CAD build for the part. Positions are in the model's coordinates, mm. A direction names the side the tool comes from. Round coordinates to 2 decimals unless told otherwise and drop trailing zeros. Loops run counter-clockwise (first coordinate to the right, second up) from the corner with the lowest first, then second, coordinate; pieces in that order, holes last. Notation, with made-up numbers: M 23,-35 L 43,-35 A14 ccw 43,-29 Z; hole C 62,20.5 d8. An arc over 180 degrees is marked long. Use a Markdown table: item, result. Add a question column.
(1) Which spindle directions (+Z, -Z, +X, -X, +Y, -Y) get a long thin tool onto all of the face, cutting with end or side? Do faces 4 (the face through (18, 91, 3)), 5 (the face through (8, -2, 3)), 6 (the face through (12.72, 107.75, 2.46)). Say none if no direction does.
(2) Band-saw the part on A-A, the plane y = 95. Write the cut outline in (x, z).
(3) Band-saw the part on D-D, the plane y = 70. Write the cut outline in (x, z), and give its area (3 significant figures).
(4) Flat gauge pins, fed straight in: P1, Ø13, axis at x = 16, y = 65, coming from the -Z side; P2, Ø0.9, axis at y = 105, z = 1.5, coming from the +X side. Where does each tip first touch, or does it go through?
(5) Two-plate mould, pull along Y, no slides. Class faces 1 (the face through (12.78, 102.25, 2.46)), 2 (the face through (11, 56, 0)), 3 (the face through (17.4, 111.43, 2.46)): released by +Y, released by -Y, zero draft, split by the parting line, or undercut.
(6) Band-saw the part on B-B, the plane x = 10. Write the cut outline in (y, z), and give its area (3 significant figures).
(7) Band-saw the part on C-C, the plane z = 1.45. Give the number of separate pieces and of enclosed holes in the cut face, and give its area (3 significant figures).
(8) Wall check: L1, parallel to Y at x = 10, z = 2.45; L2, parallel to Y at x = 2.5, z = 1.65; L3, parallel to Y at x = 4.25, z = 2.4. Give the ranges that are in metal, low to high.
from build123d import *

# Parameters (mm, degrees)
SKETCH1_W           = 24
SKETCH1_H           = 110
SKETCH1_R           = 4
SKETCH1_R_2         = 1.5
BOSS_EXTRUDE1_DEPTH = 5
SKETCH2_W           = 6
SKETCH2_H           = 37
SKETCH2_H_2         = 17
CUT_EXTRUDE1_DEPTH  = 113.698713391
BOSS_EXTRUDE2_DEPTH = 5
SKETCH4_R           = 1.5
SKETCH4_W           = 5
SKETCH4_H           = 10
CUT_EXTRUDE2_DEPTH  = 115.651646303
FILLET1_R           = 2
FILLET2_R           = 8


with BuildPart() as part:
    # Sketch1 → Boss-Extrude1 (new body)
    with BuildSketch(Plane.XY):
        with Locations((12, 55)):
            Rectangle(SKETCH1_W, SKETCH1_H)
        with Locations((16, 65)):
            Circle(SKETCH1_R, mode=Mode.SUBTRACT)
        with Locations((16, 25)):
            Circle(SKETCH1_R, mode=Mode.SUBTRACT)
        with Locations((10, 12)):
            Circle(SKETCH1_R_2, mode=Mode.SUBTRACT)
        with Locations((10, 95)):
            Circle(SKETCH1_R_2, mode=Mode.SUBTRACT)
        with BuildLine():
            Line((4, 103.5), (4, 106.5))
            ThreePointArc((4, 106.5), (5.25, 107.75), (6.5, 106.5))
            Line((6.5, 106.5), (6.5, 103.5))
            ThreePointArc((6.5, 103.5), (5.25, 102.25), (4, 103.5))
        make_face(mode=Mode.SUBTRACT)
        with BuildLine():
            Line((11.5, 103.5), (11.5, 106.5))
            ThreePointArc((11.5, 106.5), (12.75, 107.75), (14, 106.5))
            Line((14, 106.5), (14, 103.5))
            ThreePointArc((14, 103.5), (12.75, 102.25), (11.5, 103.5))
        make_face(mode=Mode.SUBTRACT)
    extrude(amount=BOSS_EXTRUDE1_DEPTH)

    # Sketch2 → Cut-Extrude1 (cut, through all)
    with BuildSketch(Plane.XY.offset(5)):
        with Locations((21, 91.5)):
            Rectangle(SKETCH2_W, SKETCH2_H)
        with Locations((21, 8.5)):
            Rectangle(SKETCH2_W, SKETCH2_H_2)
    extrude(amount=-CUT_EXTRUDE1_DEPTH, mode=Mode.SUBTRACT)

    # Sketch3 → Boss-Extrude2 (add)
    with BuildSketch(Plane.XY.offset(5)):
        Polygon((18, -2), (18, 0), (0, 0), (0, 110), (18, 110), (18, 112), (-2, 112), (-2, -2), align=None)
    extrude(amount=-BOSS_EXTRUDE2_DEPTH)

    # Sketch4 → Cut-Extrude2 (cut, through all)
    with BuildSketch(Plane.XY.offset(5)):
        with Locations((2.5, 20)):
            Circle(SKETCH4_R)
        with Locations((2.5, 70)):
            Circle(SKETCH4_R)
        with Locations((2.5, 5)):
            Rectangle(SKETCH4_W, SKETCH4_H)
        with Locations((2.5, 85)):
            Rectangle(SKETCH4_W, SKETCH4_H)
        with Locations((2.5, 45)):
            Rectangle(SKETCH4_W, SKETCH4_H)
    extrude(amount=-CUT_EXTRUDE2_DEPTH, mode=Mode.SUBTRACT)

    # Fillet1
    fillet1_edges = [part.edges().sort_by_distance(p)[0] for p in [
        (18, 112, 2.5),
        (-2, 112, 2.5),
        (-2, -2, 2.5),
        (18, -2, 2.5),
    ]]
    fillet(fillet1_edges, radius=FILLET1_R)

    # Fillet2
    # the kernel refuses this fillet: 8 mm, written as the material it takes off along each edge
    with BuildSketch(Plane(origin=(24, 17, 24.364916731), x_dir=(0, 1, 0), z_dir=(0, 0, -1))) as fillet2_piece_1:
        with BuildLine():
            CenterArc((7.745966692, -8), FILLET2_R, 90, 75.522487814)
            Line((0, -6), (-0.154919334, -5.96))
            ThreePointArc((-0.154919334, -5.96), (-0.16, -3), (-0.16, 0))
            Line((-0.16, 0), (0, 0.16))
            Line((0, 0.16), (7.745966692, 0.16))
            Line((7.745966692, 0.16), (7.745966692, 0))
        make_face()
    extrude(amount=43.729833462, mode=Mode.SUBTRACT)
    with BuildSketch(Plane(origin=(24, 73, 24.364916731), x_dir=(-1, 0, 0), z_dir=(0, 0, -1))) as fillet2_piece_2:
        with BuildLine():
            CenterArc((8, -7.745966692), FILLET2_R, 104.477512186, 75.522487814)
            Line((0, -7.745966692), (-0.16, -7.745966692))
            Line((-0.16, -7.745966692), (-0.16, 0))
            Line((-0.16, 0), (0, 0.16))
            ThreePointArc((0, 0.16), (3, 0.16), (5.96, 0.154919334))
            Line((5.96, 0.154919334), (6, 0))
        make_face()
    extrude(amount=43.729833462, mode=Mode.SUBTRACT)


solid = part.part
Return value:
| question | item | result |
|---|---|---|
| 1 | face 4 | +Z, -Z, +X, +Y |
| 1 | face 5 | +Z, -Z, +X, -X, -Y |
| 1 | face 6 | +Z, -Z |
| 2 | outline | M -2,0 L 8.5,0 L 8.5,5 L -2,5 Z; M 11.5,0 L 18,0 L 18,5 L 11.5,5 Z |
| 3 | outline | M -2,0 L 1,0 L 1,5 L -2,5 Z; M 4,0 L 22.44,0 L 22.44,5 L 4,5 Z |
| 3 | area | 107 mm^2 |
| 4 | P1 | z = 0 |
| 4 | P2 | x = 18 |
| 5 | face 1 | undercut |
| 5 | face 2 | zero draft |
| 5 | face 3 | released by +Y |
| 6 | outline | M -2,0 L 10.5,0 L 10.5,5 L -2,5 Z; M 13.5,0 L 93.5,0 L 93.5,5 L 13.5,5 Z; M 96.5,0 L 112,0 L 112,5 L 96.5,5 Z |
| 6 | area | 540 mm^2 |
| 7 | separate pieces | 1 |
| 7 | enclosed holes | 11 |
| 7 | area | 2,280 mm^2 |
| 8 | L1 | -2 to 10.5, 13.5 to 93.5, 96.5 to 112 |
| 8 | L2 | -2 to 0, 10 to 18.5, 21.5 to 40, 50 to 68.5, 71.5 to 80, 90 to 112 |
| 8 | L3 | -2 to 0, 10 to 40, 50 to 80, 90 to 102.75, 107.25 to 112 |
